Verification items for the finished model (mm, model axes). Coordinates: 2 decimals unless noted, no trailing zeros. Loops run counter-clockwise (first coordinate to the right, second up) from the corner with the lowest first, then second, coordinate; pieces in that order, holes last. Notation, with made-up numbers: M 17,11.25 L 62,11.25 A8 cw 62,20.25 Z; hole C 88,2 d10. An arc over 180 degrees is marked long. Write item = value, one per line. Start each with the question number.
```python
from build123d import *

# Parameters (mm, degrees)
F0_W     = 550
F0_H     = 550
F1_DEPTH = 19
F2_W     = 450
F2_H     = 320
F3_DEPTH = 25
F5_D     = 3
F4_W     = 44
F4_H     = 44
F4_W_2   = 22
F6_DEPTH = 25
F7_R     = 8


with BuildPart() as f1:
    # F0 (on Top) → F1 (new body)
    with BuildSketch(Plane.XY):
        Rectangle(F0_W, F0_H)
    extrude(amount=F1_DEPTH)

    # F2 (on face) → F3 (cut)
    with BuildSketch(Plane.XY.offset(19)):
        Rectangle(F2_W, F2_H)
    extrude(amount=-F3_DEPTH, mode=Mode.SUBTRACT)

    # F5 (through all)
    with Locations(Plane.XY.offset(19)):
        with Locations((220, -255), (220, -205), (170, -205), (170, -255), (-220, -205), (-220, -255), (-170, -255), (-25, -205), (-25, -255), (25, -255), (25, -205), (-170, -205)):
            Hole(F5_D / 2)

    # F4 (on face) → F6 (cut)
    with BuildSketch(Plane.XY.offset(19)):
        with Locations((195, -230)):
            Rectangle(F4_W, F4_H)
        with Locations((-195, -230)):
            Rectangle(F4_W, F4_H)
        with Locations((11, -230)):
            Rectangle(F4_W_2, F4_H)
        with Locations((-11, -230)):
            Rectangle(F4_W_2, F4_H)
    extrude(amount=-F6_DEPTH, mode=Mode.SUBTRACT)

    # F7
    f7_edges = [f1.edges().sort_by_distance(p)[0] for p in [
        (173, -208, 9.5),
        (217, -208, 9.5),
        (173, -252, 9.5),
        (217, -252, 9.5),
        (-217, -252, 9.5),
        (-217, -208, 9.5),
        (-173, -208, 9.5),
        (-173, -252, 9.5),
        (-22, -252, 9.5),
        (22, -252, 9.5),
        (22, -208, 9.5),
        (-22, -208, 9.5),
    ]]
    fillet(f7_edges, radius=F7_R)


solid = f1.part
```
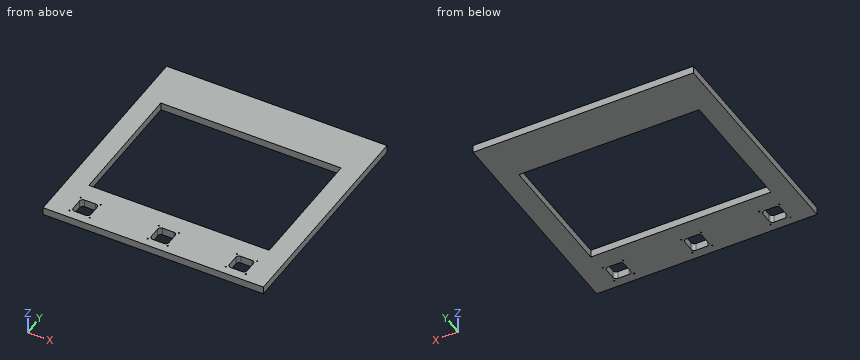
Q1. Scan lines: L1, parallel to Y at x = -25, z = 5; L2, parallel to Y at x = -192, z = 9; L3, parallel to Y at x = 129.5, z = 17. Record each from-to range of solid material in increasing order. Write a range as [from, to].
Q2. Sectioned sample at C-C on z = 4.5. Count the separate pieces of the cut face and the enclosed holes in it, plus the area to 3 significant figures.
Q3. Sectioned sample at A-A on x = 150. Record the cut outline in (y, z).
Q4. Sectioned sample at B-B on y = 30. Record the cut outline in (x, z).
Solutions:
q1.L1 = [-275, -256.5], [-253.5, -206.5], [-203.5, -160], [160, 275]
q1.L2 = [-275, -252], [-208, -160], [160, 275]
q1.L3 = [-275, -160], [160, 275]
q2.separate_pieces = 1
q2.enclosed_holes = 16
q2.area = 153,000 mm²
q3.outline = M -275,0 L -160,0 L -160,19 L -275,19 Z; M 160,0 L 275,0 L 275,19 L 160,19 Z
q4.outline = M -275,0 L -225,0 L -225,19 L -275,19 Z; M 225,0 L 275,0 L 275,19 L 225,19 Z
